Part print with two shaded views. Sizes in mm from the minimum x, y, z corner. A direction names the side the tool comes from. Round coordinates to 2 decimals unless told otherwise and drop trailing zeros. Order: outer loops, then holes, each group sorted by start corner. A loop starts at its lowest first (then second) coordinate and runs counter-clockwise, first axis right, second up. Notation, with made-up numbers: M 58.5,83 L 68.5,83 A18 ccw 68.5,104 Z; hole C 47.5,17 d6. An arc over 180 degrees is marked long. Put each result on its own line as item: value.
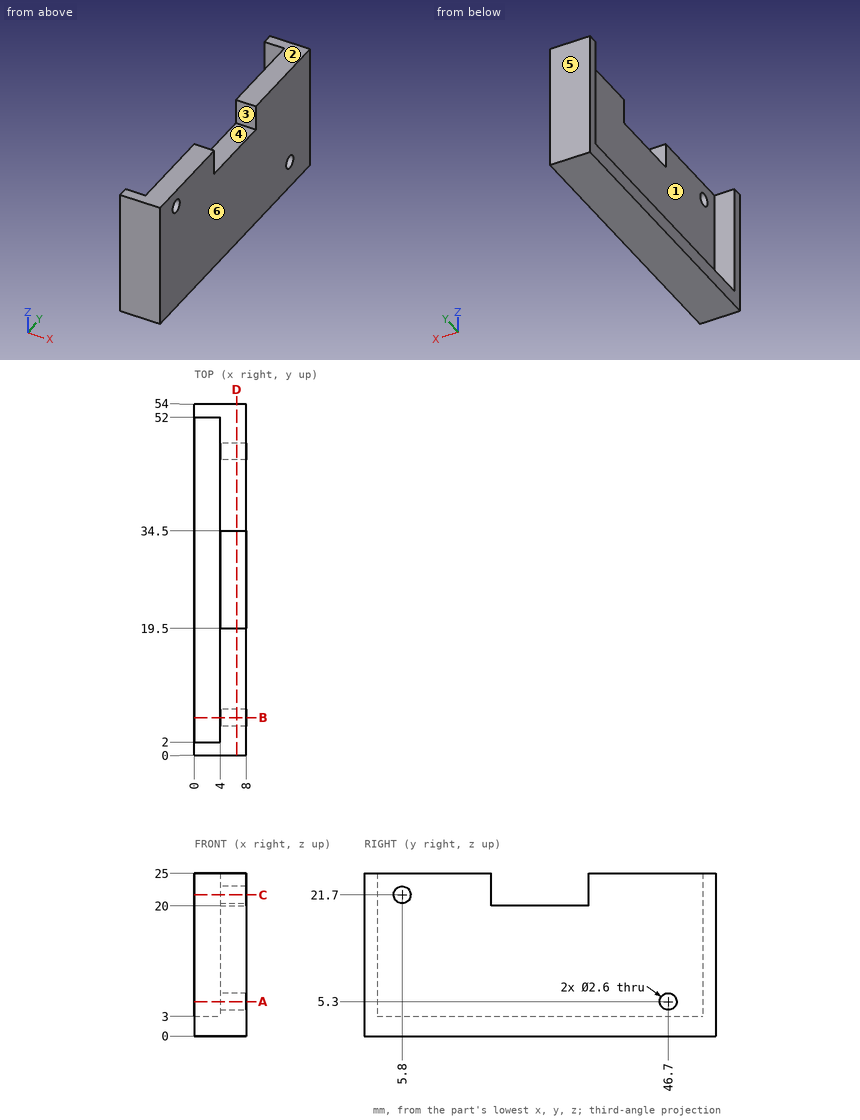
Item 1: Pin check, flat tips, straight feed: P1, Ø6.5, axis at y = 19.5, z = 9, coming from the -X side; P2, Ø2, axis at x = 6, y = 24.5, coming from the +Z side; P3, Ø1.2, axis at x = 2, y = 14.5, coming from the +Z side. Stop position of each tip, or through.
Answers below:
P1: x = 4
P2: z = 20
P3: z = 3
Item 2: Mould opens along Y. For the marked faces 4, 5 and 6 say: pulls with the +Y half, pulls with the -Y half, needs draft (parallel to the pull), parting line crosses it, or undercut.
Answers below:
face 4: undercut
face 5: pulls with the +Y half
face 6: needs draft
Item 3: Band-saw the part on D-D on x = 6.5. Give the cut face in (y, z).
Answers below:
outline: M 0,0 L 54,0 L 54,25 L 34.5,25 L 34.5,20 L 19.5,20 L 19.5,25 L 0,25 Z; hole C 5.8,21.7 d2.6; hole C 46.7,5.3 d2.6
Item 4: Band-saw the part on A-A on z = 5.3. Give the cut face in (x, y).
Answers below:
outline: M 0,0 L 8,0 L 8,45.4 L 4,45.4 L 4,2 L 0,2 Z; M 0,52 L 4,52 L 4,48 L 8,48 L 8,54 L 0,54 Z
Item 5: Band-saw the part on C-C on z = 21.7. Give the cut face in (x, y).
Answers below:
outline: M 0,0 L 8,0 L 8,4.5 L 4,4.5 L 4,2 L 0,2 Z; M 0,52 L 4,52 L 4,34.5 L 8,34.5 L 8,54 L 0,54 Z; M 4,7.1 L 8,7.1 L 8,19.5 L 4,19.5 Z
Item 6: Probe line 1 along Y through (x, z) = (6.5, 21.7); line 2 along Y through (x, z) = (2.5, 4.25); line 3 along Y through (x, z) = (5.9, 5.3). List the from-to ranges inside material, lowest first. Write a range as [from, to].
Answers below:
line 1: [0, 4.5], [7.1, 19.5], [34.5, 54]
line 2: [0, 2], [52, 54]
line 3: [0, 45.4], [48, 54]
Item 7: Tool access for the marked faces 1, 2 and 3: list every direction of +Z, -Z, +X, -X, +Y, -Y with a clear straight run to the whole face (end or side of a thin tool).
Answers below:
face 1: +Z, -X
face 2: +Z, +X, -X, +Y, -Y
face 3: +Z, +X, -X
Item 8: Band-saw the part on B-B on y = 5.8. Give the cut face in (x, z), and give its area (3 significant figures).
Answers below:
outline: M 0,0 L 8,0 L 8,20.4 L 4,20.4 L 4,3 L 0,3 Z; M 4,23 L 8,23 L 8,25 L 4,25 Z
area: 102 mm²
